from build123d import *

# Parameters (mm, degrees)
EXTRUDE_1_DEPTH = 3


with BuildPart() as part:
    # Эскиз1 → Бобышка-Вытянуть1 (new body)
    with BuildSketch(Plane(origin=(0, 0, 0), x_dir=(1, 0, 0), z_dir=(0, 1, 0))):
        Polygon((4.6, 70), (4.6, 73), (10, 73), (10, 70), (14.6, 70), (14.6, 73), (20, 73), (20, 70), (24.6, 70), (24.6, 73), (30, 73), (30, 70), (34.6, 70), (34.6, 73), (40, 73), (40, 70), (44.6, 70), (44.6, 73), (50, 73), (50, 70), (54.6, 70), (54.6, 73), (60, 73), (60, 70), (64.6, 70), (64.6, 73), (70, 73), (70, 70), (74.6, 70), (74.6, 73), (80, 73), (80, 70), (84.6, 70), (84.6, 73), (90, 73), (90, 70), (94.6, 70), (94.6, 73), (100, 73), (100, 70), (104.6, 70), (104.6, 73), (110, 73), (110, 70), (114.6, 70), (114.6, 73), (120, 73), (120, 70), (124.6, 70), (124.6, 73), (130, 73), (130, 70), (134.6, 70), (134.6, 73), (140, 73), (140, 70), (144.6, 70), (144.6, 73), (150, 73), (150, 70), (154.6, 70), (154.6, 73), (160, 73), (160, 70), (168, 70), (168, 65), (165, 65), (165, 60), (168, 60), (168, 55), (165, 55), (165, 50), (168, 50), (168, 45), (165, 45), (165, 40), (168, 40), (168, 35), (165, 35), (165, 30), (168, 30), (168, 25), (165, 25), (165, 20), (168, 20), (168, 15), (165, 15), (165, 10), (168, 10), (168, 5), (165, 5), (165, 0), (160, 0), (160, -3), (154.6, -3), (154.6, 0), (150, 0), (150, -3), (144.6, -3), (144.6, 0), (140, 0), (140, -3), (134.6, -3), (134.6, 0), (130, 0), (130, -3), (124.6, -3), (124.6, 0), (120, 0), (120, -3), (114.6, -3), (114.6, 0), (110, 0), (110, -3), (104.6, -3), (104.6, 0), (100, 0), (100, -3), (94.6, -3), (94.6, 0), (90, 0), (90, -3), (84.6, -3), (84.6, 0), (80, 0), (80, -3), (74.6, -3), (74.6, 0), (70, 0), (70, -3), (64.6, -3), (64.6, 0), (60, 0), (60, -3), (54.6, -3), (54.6, 0), (50, 0), (50, -3), (44.6, -3), (44.6, 0), (40, 0), (40, -3), (34.6, -3), (34.6, 0), (30, 0), (30, -3), (24.6, -3), (24.6, 0), (20, 0), (20, -3), (14.6, -3), (14.6, 0), (10, 0), (10, -3), (4.6, -3), (4.6, 0), (0, 0), (0, 5), (-3, 5), (-3, 10), (0, 10), (0, 15), (-3, 15), (-3, 20), (0, 20), (0, 25), (-3, 25), (-3, 30), (0, 30), (0, 35), (-3, 35), (-3, 40), (0, 40), (0, 45), (-3, 45), (-3, 50), (0, 50), (0, 55), (-3, 55), (-3, 60), (0, 60), (0, 65), (-3, 65), (-3, 70), (0, 70), align=None)
    extrude(amount=EXTRUDE_1_DEPTH)


solid = part.part
Work out the finished part from the listing and answer in its coordinate system (mm). A direction names the side the tool comes from. Coordinates: 2 decimals unless noted, no trailing zeros. Write each loop counter-clockwise with the first axis right and the second up, starting at its lowest first coordinate (ties: lowest second). Pieces come first, ordered by that corner, then holes. Notation, with made-up numbers: (24, -4) - (66, -4) arc R28 cw to (66, 14) - close; hole circle Ø6 at (88.25, 45). An arc over 180 degrees is marked (long way). One line per question, with ' | ' between items.
1) Find section B-B, the plane z = -53.5. Determine the outline of the cut face in (x, y), and give its area (3 significant figures).
Checks:
outline: (0, 0) - (165, 0) - (165, 3) - (0, 3) - close | area: 495 mm2
2) Flat-ended cylindrical pins translate along their axes: P1, Ø1.5, axis at x = -1.5, y = 1.5, coming from the -Z side; P2, Ø5, axis at x = 123.5, z = -41, coming from the -Y side; P3, Ø0.9, axis at y = 1.5, z = -71, coming from the +X side; P4, Ø0.9, axis at y = 1.5, z = -71, coming from the -X side. Find the tip coordinate at first contact, or state that the pin passes through.
Checks:
P1: z = -70 | P2: y = 0 | P3: x = 160 | P4: x = 4.6
3) Find section A-A, the plane x = 42. Determine the outline of the cut face in (y, z).
Checks:
outline: (0, -70) - (3, -70) - (3, 0) - (0, 0) - close
4) Consider probe 1 along Z at (x, y) = (11.5, 1.95); probe 2 along X at (y, z) = (2.3, -42). Determine where each line is inside the solid, lowest interval first. Write a range as [from, to].
Checks:
probe 1: [-70, 0] | probe 2: [0, 165]
5) The mould has two halves that part along Z. Classify faces 1 (the face through (-1, 1, -15)), 2 (the face through (112, 1, 0)), 3 (the face through (164, 1, -70)), 4 (the face through (70, 1, -72)): +Z half, -Z half, draft (parallel to the pull), parting line (faces both ways), or undercut.
Checks:
face 1: undercut | face 2: +Z half | face 3: -Z half | face 4: draft
6) For faces 5 (the face through (4.6, 1, 2)), 6 (the face through (132, 1, -70)), 7 (the face through (167, 1, -15)), 8 (the face through (94.6, 1, 2)), determine the directions among +Z, -Z, +X, -X, +Y, -Y from which every point of the face is accessible in a straight line to the end or side of a thin tool.
Checks:
face 5: +Z, -X, +Y, -Y | face 6: -Z, +Y, -Y | face 7: +X, +Y, -Y | face 8: +Z, +Y, -Y
